Source: three-view drawing plus pictorial views. Frame: mm from the lowest corner of the part. Give positions to 0.01 mm unless a question says otherwise; leave off trailing zeros. Order: outer loops, then holes, each group sorted by start corner. A loop starts at its lowest first (then second) coordinate and runs counter-clockwise, first axis right, second up. Notation, with made-up numbers: (77, 10) -> (110, 10) arc R21 cw to (110, 22) -> close; hole circle Ø3 at (13, -22). An arc over 180 degrees is marked (long way). Use a Markdown table: item, result. Add a question column.
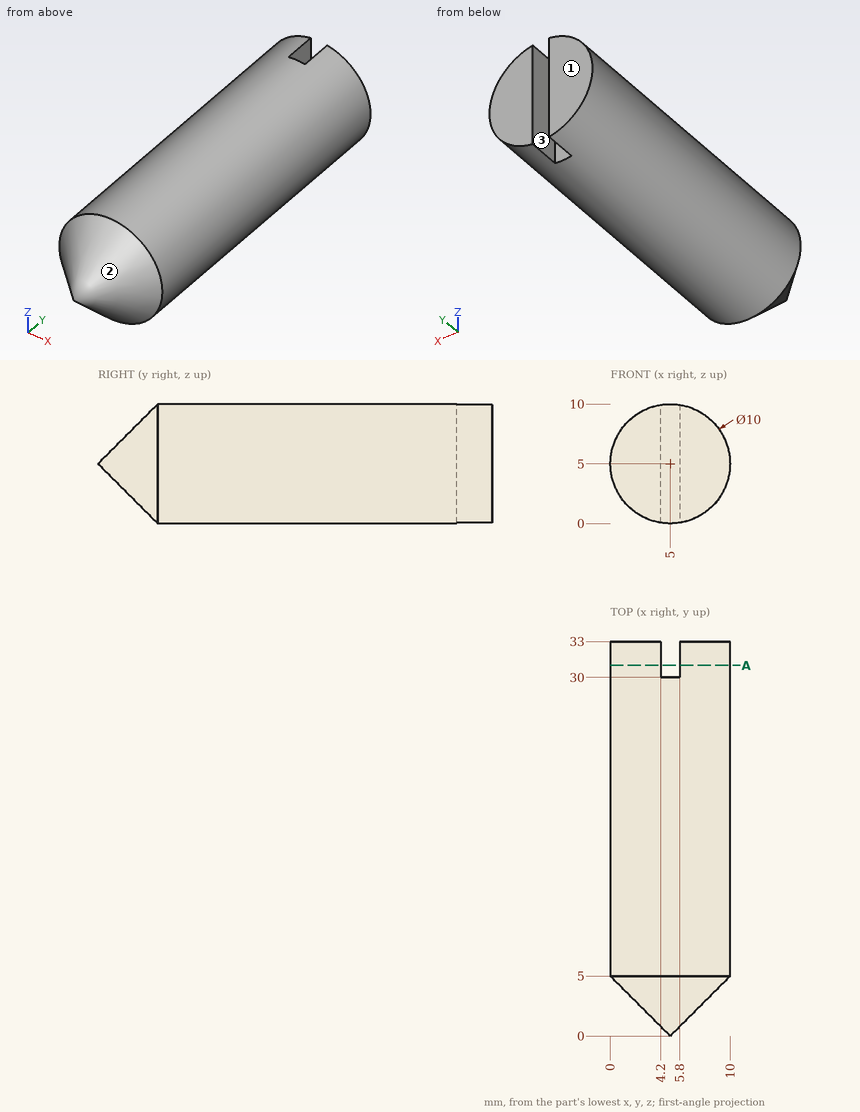
Q1. Ray query, line 1 (X direction, y = 29, z = 5.25); line 2 (Z direction, x = 7.25, y = 16). Return the intervals inside material, ascending.
Q2. Draft query along X for the marked faces 1, 2 and 3. Return one class per face: +X half, -X half, draft (parallel to the pull), parting line (faces both ways), or undercut.
Q3. Section query A-A (y = 31). Return loops of the section in (x, z).
Q4. First-contact query: pin 1 (1.5 mm diameter, centred on x = 8.5, y = 8.5, fed in from +Z); pin 2 (1.5 mm diameter, centred on y = 32, z = 7, fed in from +X); pin 3 (2.5 mm diameter, centred on y = 32, z = 7.5, fed in from -X). Flat tips, straight axial feed; report the tip coordinate or a pass-through.
Solution:
| question | item | result |
|---|---|---|
| 1 | line 1 | x = 0.01 to 9.99 |
| 1 | line 2 | z = 0.53 to 9.47 |
| 2 | face 1 | draft |
| 2 | face 2 | parting line |
| 2 | face 3 | undercut |
| 3 | outline | (4.2, 0.06) -> (4.2, 9.94) arc R5 ccw to start; (5.8, 0.06) arc R5 ccw to (5.8, 9.94) -> close |
| 4 | pin 1 | stops at z = 9.18 |
| 4 | pin 2 | stops at x = 9.84 |
| 4 | pin 3 | stops at x = 0.16 |
